from build123d import *

# Parameters (mm, degrees)
F0_W     = 381
F0_H     = 152.4
F1_DEPTH = 1.5875
F2_R     = 38.1
F3_DEPTH = 3.175
F4_R     = 38.1
F5_DEPTH = 3.175
F6_R     = 38.1
F7_DEPTH = 3.175


with BuildPart() as f1:
    # F0 (on Front) → F1 (new body, symmetric)
    with BuildSketch(Plane.XZ):
        Rectangle(F0_W, F0_H)
    extrude(amount=F1_DEPTH, both=True)

    # F2 (on face) → F3 (cut)
    with BuildSketch(Plane.XZ.offset(1.5875)):
        Circle(F2_R)
    extrude(amount=-F3_DEPTH, mode=Mode.SUBTRACT)

    # F4 (on face) → F5 (cut)
    with BuildSketch(Plane.XZ.offset(1.5875)):
        with Locations((-114.3, 0)):
            Circle(F4_R)
    extrude(amount=-F5_DEPTH, mode=Mode.SUBTRACT)

    # F6 (on face) → F7 (cut)
    with BuildSketch(Plane.XZ.offset(1.5875)):
        with Locations((114.3, 0)):
            Circle(F6_R)
    extrude(amount=-F7_DEPTH, mode=Mode.SUBTRACT)


solid = f1.part
Geometry: final body of the model. Coordinates: model frame, mm. Give positions to 0.01 mm unless a question says otherwise; leave off trailing zeros. Write each loop counter-clockwise with the first axis right and the second up, starting at its lowest first coordinate (ties: lowest second). Pieces come first, ordered by that corner, then holes. Notation, with made-up numbers: (25, 43) -> (79, 43) arc R33 cw to (79, 78) -> close; hole circle Ø8 at (46, 76). An arc over 180 degrees is marked (long way). Answer in a Markdown table with one row per item.
(1) Section query C-C on y = 0.95. Return loops of the section in (x, z), then the cut area to 3 significant figures.
Answers below:
| item | result |
|---|---|
| outline | (-190.5, -76.2) -> (190.5, -76.2) -> (190.5, 76.2) -> (-190.5, 76.2) -> close; hole circle Ø76.2 at (-114.3, 0); hole circle Ø76.2 at (0, 0); hole circle Ø76.2 at (114.3, 0) |
| area | 44,400 mm^2 |
(2) Section query A-A on z = 0. Return loops of the section in (x, y).
Answers below:
| item | result |
|---|---|
| outline | (-190.5, -1.59) -> (-152.4, -1.59) -> (-152.4, 1.59) -> (-190.5, 1.59) -> close; (-76.2, -1.59) -> (-38.1, -1.59) -> (-38.1, 1.59) -> (-76.2, 1.59) -> close; (38.1, -1.59) -> (76.2, -1.59) -> (76.2, 1.59) -> (38.1, 1.59) -> close; (152.4, -1.59) -> (190.5, -1.59) -> (190.5, 1.59) -> (152.4, 1.59) -> close |
(3) Section query D-D on z = 20. Return loops of the section in (x, y).
Answers below:
| item | result |
|---|---|
| outline | (-190.5, -1.59) -> (-146.73, -1.59) -> (-146.73, 1.59) -> (-190.5, 1.59) -> close; (-81.87, -1.59) -> (-32.43, -1.59) -> (-32.43, 1.59) -> (-81.87, 1.59) -> close; (32.43, -1.59) -> (81.87, -1.59) -> (81.87, 1.59) -> (32.43, 1.59) -> close; (146.73, -1.59) -> (190.5, -1.59) -> (190.5, 1.59) -> (146.73, 1.59) -> close |
(4) Draft query along X for faces 1 (the cylindrical face through (-30.235, -0.022, -23.183)), 2 (the flat face through (-45, 1.588, 1)). Return one class per face: +X half, -X half, draft (parallel to the pull), parting line (faces both ways), or undercut.
Answers below:
| item | result |
|---|---|
| face 1 | undercut |
| face 2 | draft |
(5) Ray query, line 1 along X through (y, z) = (0.7, 0.5); line 2 along Z through (x, y) = (0, -0.55); line 3 along X through (y, z) = (0.7, 13). Return the intervals inside material, ascending. Write a range as [from, to].
Answers below:
| item | result |
|---|---|
| line 1 | [-190.5, -152.4], [-76.2, -38.1], [38.1, 76.2], [152.4, 190.5] |
| line 2 | [-76.2, -38.1], [38.1, 76.2] |
| line 3 | [-190.5, -150.11], [-78.49, -35.81], [35.81, 78.49], [150.11, 190.5] |
(6) Section query B-B on x = 114.3. Return loops of the section in (y, z), then the cut area to 3 significant figures.
Answers below:
| item | result |
|---|---|
| outline | (-1.59, -76.2) -> (1.59, -76.2) -> (1.59, -38.1) -> (-1.59, -38.1) -> close; (-1.59, 38.1) -> (1.59, 38.1) -> (1.59, 76.2) -> (-1.59, 76.2) -> close |
| area | 242 mm^2 |
